```python
from build123d import *

# Parameters (mm, degrees)
SKETCH1_R          = 30
BASE_FLANGE1_DEPTH = 3
EDGE_FLANGE1_START = -75
EDGE_FLANGE1_DEPTH = 140
EDGE_FLANGE2_START = -75
EDGE_FLANGE2_DEPTH = 140
EDGE_FLANGE3_DEPTH = 130
SKETCH23_R         = 30
CUT_EXTRUDE1_DEPTH = 10
SKETCH24_R         = 30
CUT_EXTRUDE2_DEPTH = 10
FILLET1_R          = 10


# Read off the part's stored shape, not the designer's step: Edge-Flange1, Edge-Flange2
# Sheet-metal steps are written as plain solids
with BuildPart() as part:
    # Sketch1 → Base-Flange1 (new body)
    with BuildSketch(Plane(origin=(0, 0, 0), x_dir=(1, 0, 0), z_dir=(0, 1, 0))):
        with BuildLine():
            Line((65, -75), (-65, -75))
            ThreePointArc((-65, -75), (-67.928932188, -67.928932188), (-75, -65))
            Line((-75, -65), (-75, 75))
            Line((-75, 75), (75, 75))
            Line((75, 75), (75, -65))
            ThreePointArc((75, -65), (67.928932188, -67.928932188), (65, -75))
        make_face()
        with Locations(Location((0, 0, 0), (0, 0, 270))):
            Circle(SKETCH1_R, mode=Mode.SUBTRACT)
    extrude(amount=-BASE_FLANGE1_DEPTH)

    # Edge-Flange1 outline → Edge-Flange1 (add)
    with BuildSketch(Plane.XY.offset(EDGE_FLANGE1_START)):
        with BuildLine():
            Line((-188.066017178, 103.066017178), (-83.094424801, -1.905575199))
            ThreePointArc((-83.094424801, -1.905575199), (-81.882184516, -2.715568261), (-80.452249603, -3))
            Line((-80.452249603, -3), (-75, -3))
            Line((-75, -3), (-75, 0))
            Line((-75, 0), (-80.452249603, 0))
            ThreePointArc((-80.452249603, 0), (-80.734134219, 0.056070336), (-80.973104458, 0.215745145))
            Line((-80.973104458, 0.215745145), (-185.944696834, 105.187337522))
            Line((-185.944696834, 105.187337522), (-188.066017178, 103.066017178))
        make_face()
    extrude(amount=EDGE_FLANGE1_DEPTH)

    # Edge-Flange2 outline → Edge-Flange2 (add)
    with BuildSketch(Plane.XY.offset(EDGE_FLANGE2_START)):
        with BuildLine():
            ThreePointArc((80.452249603, -3), (81.882184516, -2.715568261), (83.094424801, -1.905575199))
            Line((83.094424801, -1.905575199), (188.066017178, 103.066017178))
            Line((188.066017178, 103.066017178), (185.944696834, 105.187337522))
            Line((185.944696834, 105.187337522), (80.973104458, 0.215745145))
            ThreePointArc((80.973104458, 0.215745145), (80.734134219, 0.056070336), (80.452249603, 0))
            Line((80.452249603, 0), (75, 0))
            Line((75, 0), (75, -3))
            Line((75, -3), (80.452249603, -3))
        make_face()
    extrude(amount=EDGE_FLANGE2_DEPTH)

    # Edge-Flange3 section (across the edge) → Edge-Flange3 (add)
    with BuildSketch(Plane(origin=(65, -3, 85), x_dir=(0, 0, -1), z_dir=(-1, 0, 0))):
        with BuildLine():
            Line((0, 0.7366), (0, 147))
            Line((0, 147), (3, 147))
            Line((3, 147), (3, 0.7366))
            ThreePointArc((3, 0.7366), (3.215745145, 0.215745145), (3.7366, 0))
            Line((3.7366, 0), (10, 0))
            Line((10, 0), (10, -3))
            Line((10, -3), (3.7366, -3))
            ThreePointArc((3.7366, -3), (1.094424801, -1.905575199), (0, 0.7366))
        make_face()
    extrude(amount=EDGE_FLANGE3_DEPTH)

    # Sketch23 → Cut-Extrude1 (cut)
    with BuildSketch(Plane(origin=(-40.378679656, -40.378679656, 0), x_dir=(0, 0, -1), z_dir=(0.7071067811865438, 0.7071067811865513, 0))):
        with Locations(Location((0, 130.861435714, 0), (0, 0, 90))):
            Circle(SKETCH23_R)
    cut_extrude1 = extrude(amount=-CUT_EXTRUDE1_DEPTH, mode=Mode.SUBTRACT)

    # Mirror1: Cut-Extrude1 across plane
    add(cut_extrude1.mirror(Plane(origin=(0, 0, 0), x_dir=(0, 0, 1), z_dir=(1, 0, 0))), mode=Mode.SUBTRACT)

    # Sketch24 → Cut-Extrude2 (cut)
    with BuildSketch(Plane.XY.offset(85)):
        with Locations((0, -75)):
            Circle(SKETCH24_R)
    extrude(amount=-CUT_EXTRUDE2_DEPTH, mode=Mode.SUBTRACT)

    # Fillet1
    fillet1_edges = [part.edges().sort_by_distance(p)[0] for p in [
        (-187.005357006, 104.12667735, -75),
        (-187.005357006, 104.12667735, 65),
        (187.005357006, 104.12667735, 65),
        (187.005357006, 104.12667735, -75),
        (65, -150, 83.5),
        (-65, -150, 83.5),
    ]]
    fillet(fillet1_edges, radius=FILLET1_R)


solid = part.part
```
Here's how the part is built. I have some questions about the finished solid (model axes, mm). A direction names the side the tool comes from. Coordinates: 2 decimals unless noted, no trailing zeros. Loops run counter-clockwise (first coordinate to the right, second up) from the corner with the lowest first, then second, coordinate; pieces in that order, holes last. Notation, with made-up numbers: (50, -4) -> (89, -4) arc R10 ccw to (89, 9) -> close; hole circle Ø11 at (27.25, 26.25). An arc over 180 degrees is marked (long way). Return JSON: item names as keys, results as strings.
1) For faces 1 (the face through (1.1, -3, -30.5)), 2 (the face through (154.191, 71.342, 9.011)), which set-ups out of +Z, -Z, +X, -X, +Y, -Y let a thin tool reach every point of the face, with its end or its side?
Results below:
{"face 1": "-Z, +X, -X, -Y", "face 2": "none"}
2) If we section it at C-C, the plane z = 0: Write out the boundary of the cut face in (x, y), then the cut area to 3 significant figures.
Results below:
{"outline": "(-188.07, 103.07) -> (-156.25, 71.25) -> (-154.12, 73.37) -> (-185.94, 105.19) -> close; (-113.82, 28.82) -> (-83.09, -1.91) arc R3.74 ccw to (-80.45, -3) -> (-30, -3) -> (-30, 0) -> (-80.45, 0) arc R0.74 cw to (-80.97, 0.22) -> (-111.7, 30.94) -> close; (30, -3) -> (80.45, -3) arc R3.74 ccw to (83.09, -1.91) -> (113.82, 28.82) -> (111.7, 30.94) -> (80.97, 0.22) arc R0.74 cw to (80.45, 0) -> (30, 0) -> close; (154.12, 73.37) -> (156.25, 71.25) -> (188.07, 103.07) -> (185.94, 105.19) -> close", "area": "844 mm²"}
3) If we section it at B-B, the plane x = 0: Write out the boundary of the cut face in (y, z), then the cut area to 3 significant figures.
Results below:
{"outline": "(-150, 82) -> (-105, 82) -> (-105, 85) -> (-150, 85) -> close; (-45, 82) -> (-3.74, 82) arc R0.74 cw to (-3, 81.26) -> (-3, 30) -> (0, 30) -> (0, 81.26) arc R3.74 ccw to (-3.74, 85) -> (-45, 85) -> close; (-3, -75) -> (0, -75) -> (0, -30) -> (-3, -30) -> close", "area": "558 mm²"}
4) If we section it at D-D, the plane x = -40: Write out the boundary of the cut face in (y, z), then the cut area to 3 significant figures.
Results below:
{"outline": "(-150, 82) -> (-3.74, 82) arc R0.74 cw to (-3, 81.26) -> (-3, -75) -> (0, -75) -> (0, 81.26) arc R3.74 ccw to (-3.74, 85) -> (-150, 85) -> close", "area": "918 mm²"}
5) Thinking about a two-plate mould opening in X: for faces 3 (the face through (134.194, 53.436, -37.091)), 4 (the face through (-184.89, 101.99, 62.15)), 5 (the face through (-1, -1, -75)), which applies, +X half, -X half, draft (parallel to the pull), parting line (faces both ways), or undercut?
Results below:
{"face 3": "undercut", "face 4": "-X half", "face 5": "draft"}
6) If we section it at A-A, the plane y = -75: Write out the boundary of the cut face in (x, z), then the cut area to 3 significant figures.
Results below:
{"outline": "(-65, 82) -> (-30, 82) -> (-30, 85) -> (-65, 85) -> close; (30, 82) -> (65, 82) -> (65, 85) -> (30, 85) -> close", "area": "210 mm²"}
7) Will these pins go through, and if not, where does the flat tip stop? pin 1 (6 mm diameter, centred on x = 46, y = -83, fed in from -Z); pin 2 (6 mm diameter, centred on x = 135.5, z = -32.5, fed in from +Y); pin 3 (5 mm diameter, centred on y = -81, z = 80, fed in from +X).
Results below:
{"pin 1": "z = 82", "pin 2": "y = 57.74", "pin 3": "x = 65"}
8) I need wall thicknesses on line 1 (Y direction, x = -18.5, z = -51.5); line 2 (Y direction, x = 0, z = 83.1); line 3 (X direction, y = -0.75, z = 0). Which ranges of each line are inside material? Lowest first, please. Write a range as from..to.
Results below:
{"line 1": "-3..0", "line 2": "-150..-105, -45..-0.48", "line 3": "-84.25..-30, 30..84.25"}
